from build123d import *

# Parameters (mm, degrees)
SKETCH2_R               = 5
BOSS_EXTRUDE1_DEPTH     = 8
SKETCH4_R               = 4.55
CUT_EXTRUDE1_DEPTH      = 7.1
CUT_EXTRUDE2_DEPTH      = 11.677078252
CUT_EXTRUDE2_DEPTH_BACK = 11.677078252
SKETCH12_R              = 1.9
SKETCH13_W              = 3.8
SKETCH13_H              = 2.1
CUT_EXTRUDE3_DEPTH      = 10


with BuildPart() as part:
    # Sketch2 → Boss-Extrude1 (new body)
    with BuildSketch(Plane(origin=(0, 0, 0), x_dir=(1, 0, 0), z_dir=(0, 1, 0))):
        with Locations(Location((0, 0, 0), (0, 0, 270))):
            Circle(SKETCH2_R)
    extrude(amount=BOSS_EXTRUDE1_DEPTH)

    # Sketch4 → Cut-Extrude1 (cut)
    with BuildSketch(Plane(origin=(0, 0, 0), x_dir=(1, 0, 0), z_dir=(0, 1, 0))):
        with Locations(Location((0, 0, 0), (0, 0, 270))):
            Circle(SKETCH4_R)
    extrude(amount=CUT_EXTRUDE1_DEPTH, mode=Mode.SUBTRACT)

    # Sketch12 → Cut-Extrude2 (cut, two sides: drawn at the far end of the back side and taken through both)
    with BuildSketch(Plane.XY.offset(-CUT_EXTRUDE2_DEPTH_BACK)):
        with Locations((0, 2.1)):
            Circle(SKETCH12_R)
    extrude(amount=CUT_EXTRUDE2_DEPTH + CUT_EXTRUDE2_DEPTH_BACK, mode=Mode.SUBTRACT)

    # Sketch13 → Cut-Extrude3 (cut)
    with BuildSketch(Plane.XY):
        with Locations((0, 1.05)):
            Rectangle(SKETCH13_W, SKETCH13_H)
    extrude(amount=-CUT_EXTRUDE3_DEPTH, mode=Mode.SUBTRACT)


solid = part.part
The model under review builds one solid part; all positions refer to its coordinate system, in mm. Give positions to 0.01 mm unless a question says otherwise; leave off trailing zeros. Loops run counter-clockwise (first coordinate to the right, second up) from the corner with the lowest first, then second, coordinate; pieces in that order, holes last. Notation, with made-up numbers: (52.5, 78) -> (100.5, 78) arc R23 cw to (100.5, 98) -> close; hole circle Ø5 at (45.25, 11.5). An arc over 180 degrees is marked (long way). Write each question's results on one line, items separated by ' | '.
1) Take a section at B-B, the plane z = 0. Give the boundary of the cut face in (x, y).
Conclusion:
outline: (-5, 0) -> (-4.55, 0) -> (-4.55, 7.1) -> (4.55, 7.1) -> (4.55, 0) -> (5, 0) -> (5, 8) -> (-5, 8) -> close
2) Insertion check: pin 1 Ø0.5 at (y, z) = (1, -4.5) entering from +X; pin 2 Ø4 at (y, z) = (2, -2.5) entering from -X; pin 3 Ø0.5 at (y, z) = (1, -4.5) entering from -X. Each pin has a flat end and moves straight along its axis. Give the tip position at first contact, or say it passes through.
Conclusion:
pin 1: stops at x = 2.63 | pin 2: stops at x = -4.97 | pin 3: stops at x = -2.63
3) Take a section at A-A, the plane x = 0. Give the boundary of the cut face in (y, z).
Conclusion:
outline: (0, 4.55) -> (0.2, 4.55) -> (0.2, 5) -> (0, 5) -> close; (4, -5) -> (8, -5) -> (8, 5) -> (4, 5) -> (4, 4.55) -> (7.1, 4.55) -> (7.1, -4.55) -> (4, -4.55) -> close
4) Take a section at D-D, the plane y = 1.5. Give the boundary of the cut face in (x, z), plus the area to 3 significant figures.
Conclusion:
outline: (-1.9, -4.62) -> (-1.9, -4.13) arc R4.55 cw to (-1.8, 4.18) -> (-1.8, 4.66) arc R5 ccw to start; (1.8, 4.18) arc R4.55 cw to (1.9, -4.13) -> (1.9, -4.62) arc R5 ccw to (1.8, 4.66) -> close | area: 10.1 mm^2
5) Take a section at C-C, the plane y = 3. Give the boundary of the cut face in (x, z), plus the area to 3 significant figures.
Conclusion:
outline: (-1.67, -4.71) -> (-1.67, -4.23) arc R4.55 cw to (-1.67, 4.23) -> (-1.67, 4.71) arc R5 ccw to start; (1.67, -4.71) arc R5 ccw to (1.67, 4.71) -> (1.67, 4.23) arc R4.55 cw to (1.67, -4.23) -> close | area: 10.4 mm^2
6) For line 1 along Z through (x, y) = (0, 5.75); line 2 along Y through (x, z) = (0, 4.6), list the stretches that pass through material, from the lowest coordinate up. Write a range as from..to.
Conclusion:
line 1: z = -5..-4.55, 4.55..5 | line 2: y = 0..0.2, 4..8
7) Draft analysis for pull direction X (two halves, no side actions). For faces 1 (the face through (-4.037, 3.5, 2.1)), 2 (the face through (-1.915, 3.944, 4.619)), 3 (the face through (0, 8, 0)), state which applies: pulls with the +X half, pulls with the -X half, needs draft (parallel to the pull), parting line crosses it, or undercut.
Conclusion:
face 1: undercut | face 2: parting line crosses it | face 3: needs draft
